Model file for the job. Use its own axes, mm. A direction names the side the tool comes from. Round coordinates to 2 decimals unless told otherwise and drop trailing zeros. Order: outer loops, then holes, each group sorted by start corner. A loop starts at its lowest first (then second) coordinate and runs counter-clockwise, first axis right, second up. Notation, with made-up numbers: (13, 67.25) -> (53, 67.25) arc R18 ccw to (53, 88.25) -> close; hole circle Ø1 at (24.25, 32.5). An arc over 180 degrees is marked (long way). Use CSV: the item, a comma, the result in double quotes.
```python
from build123d import *

# Parameters (mm, degrees)
EXTRUDE_1_DEPTH     = 5
CUT_EXTRUDE_1_REACH = 93.591
SKETCH_5_R          = 4.7


# Read off the part's stored shape, not the designer's step: 高级异型孔1
with BuildPart() as part:
    # 草图1 → 凸台-拉伸1 (new, symmetric)
    with BuildSketch(Plane(origin=(10, 0, 0), x_dir=(0, 0, -1), z_dir=(1, 0, 0))):
        with BuildLine():
            Line((-18, 80), (-18, 90))
            Line((-18, 90), (-24, 90))
            Line((-24, 90), (-24, 84.649110641))
            ThreePointArc((-24, 84.649110641), (-32, 72), (-24, 59.350889359))
            Line((-24, 59.350889359), (-24, 54))
            Line((-24, 54), (-18, 54))
            Line((-18, 54), (-18, 64))
            ThreePointArc((-18, 64), (-26, 72), (-18, 80))
        make_face()
    extrude(amount=EXTRUDE_1_DEPTH, both=True)

    # 高级异型孔1 outline → 高级异型孔1 (revolve, cut)
    with BuildSketch(Plane(origin=(10, 59, 0), x_dir=(1, 0, 0), z_dir=(0, -1, 0))):
        Polygon((0, 18), (2.25, 18), (2.25, 21.55), (4.7, 24), (0, 24), align=None)
    revolve(axis=Axis((10, 59, 0), (0, 0, 1)), mode=Mode.SUBTRACT)

    # Other 1 2 outline → Other 1 2 (revolve, cut)
    with BuildSketch(Plane(origin=(10, 85, 0), x_dir=(1, 0, 0), z_dir=(0, -1, 0))):
        Polygon((0, 18), (2.25, 18), (2.25, 21.55), (4.7, 24), (0, 24), align=None)
    revolve(axis=Axis((10, 85, 0), (0, 0, 1)), mode=Mode.SUBTRACT)

    # 草图5 → 切除-拉伸1 (cut, up to next)
    with BuildSketch(Plane.XY.offset(24), mode=Mode.PRIVATE) as cut_extrude_1_sk1:
        with Locations((10, 85)):
            Circle(SKETCH_5_R)
    cut_extrude_1_tool1 = extrude(cut_extrude_1_sk1.sketch, amount=CUT_EXTRUDE_1_REACH, mode=Mode.PRIVATE) & part.part
    # 草图5 → 切除-拉伸1 (cut, up to next)
    with BuildSketch(Plane.XY.offset(24), mode=Mode.PRIVATE) as cut_extrude_1_sk2:
        with Locations((10, 59)):
            Circle(SKETCH_5_R)
    cut_extrude_1_tool2 = extrude(cut_extrude_1_sk2.sketch, amount=CUT_EXTRUDE_1_REACH, mode=Mode.PRIVATE) & part.part
    add(cut_extrude_1_tool1.solids().sort_by_distance((10, 85, 24))[0], mode=Mode.SUBTRACT)
    add(cut_extrude_1_tool2.solids().sort_by_distance((10, 59, 24))[0], mode=Mode.SUBTRACT)


solid = part.part
```
Q1. Cut at D-D (z = 22.5). Give the cut face in (x, y), plus the area to 3 significant figures.
From the geometry:
outline,"(5, 54) -> (15, 54) -> (15, 65.39) -> (5, 65.39) -> close; (5, 78.61) -> (15, 78.61) -> (15, 90) -> (5, 90) -> close; hole circle Ø6.4 at (10, 59); hole circle Ø6.4 at (10, 85)"
area,"163 mm²"
Q2. Cut at C-C (z = 20.25). Give the cut face in (x, y).
From the geometry:
outline,"(5, 54) -> (15, 54) -> (15, 64.32) -> (5, 64.32) -> close; (5, 79.68) -> (15, 79.68) -> (15, 90) -> (5, 90) -> close; hole circle Ø4.5 at (10, 59); hole circle Ø4.5 at (10, 85)"
Q3. Pin check, flat tips, straight feed: pin 1 (1 mm diameter, centred on x = 9.5, y = 77.5, fed in from +Z); pin 2 (4.5 mm diameter, centred on x = 10, y = 86.5, fed in from +Z); pin 3 (8 mm diameter, centred on y = 80, z = 30, fed in from -X); pin 4 (3.5 mm diameter, centred on x = 10, y = 59, fed in from +Z). Stop position of each tip, or through.
From the geometry:
pin 1,"stops at z = 31.08"
pin 2,"stops at z = 23.05"
pin 3,"stops at x = 5"
pin 4,"passes through"
Q4. Mould opens along Y. For faces 1 (the flat face through (11.13, 89.72, 24)), 2 (the conical face through (11.11, 56.87, 21.7)), 3 (the cylindrical face through (9.9, 80.3, 26)), 4 (the conical face through (11.11, 82.87, 21.7)) say: +Y half, -Y half, draft (parallel to the pull), parting line (faces both ways), or undercut.
From the geometry:
face 1,"draft"
face 2,"undercut"
face 3,"+Y half"
face 4,"undercut"
Q5. Cut at B-B (x = 10). Give the cut face in (y, z), plus the area to 3 significant figures.
From the geometry:
outline,"(54, 18) -> (56.75, 18) -> (56.75, 21.55) -> (54.3, 24) -> (54, 24) -> close; (61.25, 18) -> (64, 18) arc R8 cw to (80, 18) -> (82.75, 18) -> (82.75, 21.55) -> (80.3, 24) -> (80.3, 29.27) arc R14 ccw to (63.7, 29.27) -> (63.7, 24) -> (61.25, 21.55) -> close; (87.25, 18) -> (90, 18) -> (90, 24) -> (89.7, 24) -> (87.25, 21.55) -> close"
area,"168 mm²"
Q6. Which spindle directions (+Z, -Z, +X, -X, +Y, -Y) get a long thin tool onto all of the face, cutting with end or side? Do faces 5 (the flat face through (8.5, 54.3, 24)), 6 (the flat face through (11.2, 56.7, 18)), 7 (the cylindrical face through (10.1, 63.7, 26)). Say none if no direction does.
From the geometry:
face 5,"+Z, +X, -X, -Y"
face 6,"-Z, +X, -X, +Y, -Y"
face 7,"+Z, -Y"
Q7. Cut at A-A (y = 85). Give the cut face in (x, z), plus the area to 3 significant figures.
From the geometry:
outline,"(5, 18) -> (7.75, 18) -> (7.75, 21.55) -> (5.3, 24) -> (5, 24) -> close; (12.25, 18) -> (15, 18) -> (15, 24) -> (14.7, 24) -> (12.25, 21.55) -> close"
area,"27.0 mm²"
Q8. Probe line 1 along Y through (x, z) = (10, 20.6); line 2 along Y through (x, z) = (10, 20.15); line 3 along Y through (x, z) = (9.75, 25). List the from-to ranges inside material, lowest first.
From the geometry:
line 1,"y = 54 to 56.75, 61.25 to 64.43, 79.57 to 82.75, 87.25 to 90"
line 2,"y = 54 to 56.75, 61.25 to 64.29, 79.71 to 82.75, 87.25 to 90"
line 3,"y = 63.69 to 68.13, 75.87 to 80.31"
